Build history of the part. All positions in model axes, mm. Give positions to 0.01 mm unless a question says otherwise; leave off trailing zeros. Loops run counter-clockwise (first coordinate to the right, second up) from the corner with the lowest first, then second, coordinate; pieces in that order, holes last. Notation, with made-up numbers: (9.25, 1) - (35.25, 1) arc R19 ccw to (35.25, 16) - close; hole circle Ø3 at (14.5, 12). An arc over 180 degrees is marked (long way). Return JSON: item names as keys, results as strings. Group by question number.
1) Drop a flat-ended pin along its axis: pin 1 (1 mm diameter, centred on y = 2.5, z = -48, fed in from -X). Give the stop position or say it passes through.
2) Drill centre lines: probe 1 along Z at (x, y) = (65, 0.2); probe 2 along X at (y, z) = (0.95, -62); probe 3 along Z at (x, y) = (44.5, 1). Where is each one in solid material? Low to high. Write a range as from..to.
3) Slice it at D-D (x = -18). List the corners of the cut face in (y, z), and give its area (3 significant figures).
4) Slice it at B-B (z = 47.5). List the corners of the cut face in (x, y), and give its area (3 significant figures).
5) Slice it at C-C (y = 1.4). List the corners of the cut face in (x, z), and give its area (3 significant figures).
6) Slice it at A-A (x = 46.5). List the corners of the cut face in (y, z).
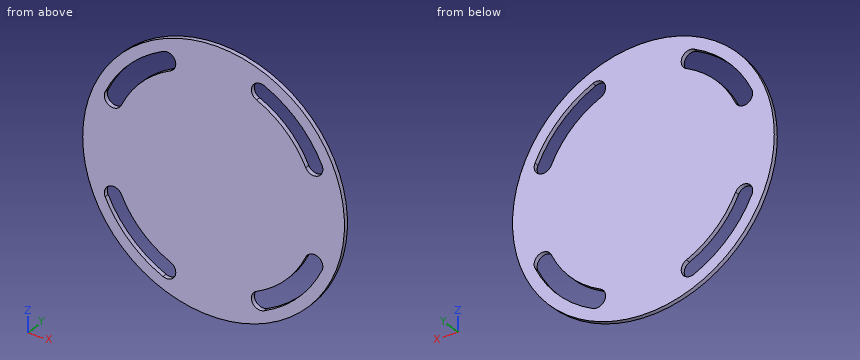
Autodesk Inventor part; units mm, degrees
ref_plane "YZ Plane" through (0, 0, 0) normal (1, 0, 0) x (0, 1, 0)
ref_plane "XZ Plane" through (0, 0, 0) normal (0, 1, 0) x (-1, 0, 0)
ref_plane "XY Plane" through (0, 0, 0) normal (0, 0, 1) x (1, 0, 0)
sketch "Sketch1" plane through (0, 0, 0) normal (0, 1, 0) x (-1, 0, 0)
  circle A0 centre (0, 0) radius 87.5
  dimension "d0" = 175
extrude "Plate1" add sketch "Sketch1" along normal blind 3
sketch "Sketch2" plane through (0, 3, 0) normal (0, 1, 0) x (1, 0, 0)
  line L0 (-40, -40) -> (40, -40) construction
  line L1 (40, -40) -> (40, 40) construction
  line L2 (40, 40) -> (-40, 40) construction
  line L3 (-40, 40) -> (-40, -40) construction
  line L4 (-40, -40) -> (40, 40) construction
  circle A0 centre (0, 0) radius 87.5
  circle A1 centre (0, 0) radius 74 construction
  circle A2 centre (-67.0668, -31.2738) radius 6
  line L5 (-67.0668, -31.2738) -> (0, 0) construction
  circle A3 centre (-31.2738, -67.0668) radius 6
  line L6 (-31.2738, -67.0668) -> (0, 0) construction
  arc A4 (-72.5046, -33.8095) -> (-33.8095, -72.5046) centre (0, 0) ccw
  arc A5 (-61.6289, -28.738) -> (-28.738, -61.6289) centre (0, 0) ccw
  point P0 (-61.6289, -28.738)
  point P1 (-28.738, -61.6289)
  dimension "d7" = 12
  dimension "d9" = 12
  dimension "d2" = 80
  dimension "d3" = 80
  dimension "d16" = 40
  dimension "d17" = 20
  dimension "d18" = 13.5
extrude "Extrusion1" cut sketch "Sketch2" against normal through all contours A2 | A2 A5 A3 A4 | A3
pattern_circular "Circular Pattern1" count 4 over 360 about axis through (0, -10, 0) along (0, 1, 0) of "Extrusion1"
equation "\"d9\" = d7"
equation "\"BendReliefWidth\" = Thickness"
equation "\"BendReliefDepth\" = 0.5 * Thickness"
equation "\"CornerReliefSize\" = 4 * Thickness"
equation "\"MinimumRemnant\" = 2 * Thickness"
equation "\"TransitionRadius\" = BendRadius"
equation "\"JacobiRadiusSize\" = BendRadius"
equation "\"GapSize\" = Thickness"
properties part number "MSC 126 flange frame" material "Stainless Steel"
Results:
{
 "1": {"pin 1": "x = -73.48"},
 "2": {"probe 1": "-58.58..-46.64, -25.64..25.64, 46.64..58.58", "probe 2": "-61.74..-50.56, -28.06..28.06, 50.56..61.74", "probe 3": "-75.34..-66.48, -51.42..51.42, 66.48..75.34"},
 "3": {"outline": "(0, -85.63) - (3, -85.63) - (3, 85.63) - (0, 85.63) - close", "area": "514 mm2"},
 "4": {"outline": "(-73.48, 0) - (-64.37, 0) - (-64.37, 3) - (-73.48, 3) - close; (-48.66, 0) - (48.66, 0) - (48.66, 3) - (-48.66, 3) - close; (64.37, 0) - (73.48, 0) - (73.48, 3) - (64.37, 3) - close", "area": "347 mm2"},
 "5": {"outline": "circle Ø175 at (0, 0); hole (-72.5, -33.81) arc R80 ccw to (-33.81, -72.5) arc R6 ccw to (-28.74, -61.63) arc R68 cw to (-61.63, -28.74) arc R6 ccw to start; hole (-72.5, 33.81) arc R6 ccw to (-61.63, 28.74) arc R68 cw to (-28.74, 61.63) arc R6 ccw to (-33.81, 72.5) arc R80 ccw to start; hole (28.74, -61.63) arc R6 ccw to (33.81, -72.5) arc R80 ccw to (72.5, -33.81) arc R6 ccw to (61.63, -28.74) arc R68 cw to start; hole (28.74, 61.63) arc R68 cw to (61.63, 28.74) arc R6 ccw to (72.5, 33.81) arc R80 ccw to (33.81, 72.5) arc R6 ccw to start", "area": "21,100 mm2"},
 "6": {"outline": "(0, -74.12) - (3, -74.12) - (3, -65.1) - (0, -65.1) - close; (0, -49.62) - (3, -49.62) - (3, 49.62) - (0, 49.62) - close; (0, 65.1) - (3, 65.1) - (3, 74.12) - (0, 74.12) - close"}
}
